from build123d import *

# Parameters (mm, degrees)
SKETCH1_W           = 50
SKETCH1_H           = 50
BOSS_EXTRUDE1_DEPTH = 3
BOSS_EXTRUDE2_DEPTH = 6
CUT_EXTRUDE1_DEPTH  = 2.1
CUT_EXTRUDE2_DEPTH  = 2.5
CUT_EXTRUDE3_DEPTH  = 3.3
SKETCH4_R           = 1.55
SKETCH4_R_2         = 1.8
SKETCH4_R_3         = 2.4
CUT_EXTRUDE4_DEPTH  = 37.482872694
CUT_EXTRUDE5_REACH  = 38.483
SKETCH5_W           = 3.1
SKETCH5_H           = 6
SKETCH5_W_2         = 6
SKETCH5_H_2         = 3.6
SKETCH5_W_3         = 4.8


with BuildPart() as part:
    # Sketch1 → Boss-Extrude1 (new body)
    with BuildSketch(Plane(origin=(0, 0, 0), x_dir=(1, 0, 0), z_dir=(0, 1, 0))):
        Rectangle(SKETCH1_W, SKETCH1_H)
    extrude(amount=BOSS_EXTRUDE1_DEPTH)

    # Sketch2 → Boss-Extrude2 (add)
    with BuildSketch(Plane(origin=(0, 3, 0), x_dir=(1, 0, 0), z_dir=(0, 1, 0))):
        Polygon((-13, 13), (-25, 13), (-25, 25), (25, 25), (25, -25), (-25, -25), (-25, -13), (-13, -13), (13, -13), (13, 13), align=None)
    extrude(amount=BOSS_EXTRUDE2_DEPTH)

    # Sketch3 → Cut-Extrude1 (cut)
    with BuildSketch(Plane(origin=(0, 3, 0), x_dir=(1, 0, 0), z_dir=(0, 1, 0))):
        Polygon((-21.5, 25), (-16.5, 25), (-16.5, 20.443375673), (-16.5, 17.556624327), (-19, 16.113248654), (-21.5, 17.556624327), (-21.5, 20.443375673), align=None)
        Polygon((-8.55, 25), (-3.45, 25), (-3.45, 20.472243186), (-3.45, 17.527756814), (-6, 16.055513627), (-8.55, 17.527756814), (-8.55, 20.472243186), align=None)
        Polygon((4.4, 25), (9.6, 25), (9.6, 20.5011107), (9.6, 17.4988893), (7, 15.9977786), (4.4, 17.4988893), (4.4, 20.5011107), align=None)
    extrude(amount=CUT_EXTRUDE1_DEPTH, mode=Mode.SUBTRACT)

    # Sketch3<3> → Cut-Extrude2 (cut)
    with BuildSketch(Plane(origin=(0, 3, 0), x_dir=(1, 0, 0), z_dir=(0, 1, 0))):
        Polygon((25, 15.75), (25, 10.25), (20.58771324, 10.25), (17.41228676, 10.25), (15.824573519, 13), (17.41228676, 15.75), (20.58771324, 15.75), align=None)
        Polygon((25, 2.8), (25, -2.8), (20.616580754, -2.8), (17.383419246, -2.8), (15.766838493, 0), (17.383419246, 2.8), (20.616580754, 2.8), align=None)
        Polygon((25, -10.15), (25, -15.85), (20.645448267, -15.85), (17.354551733, -15.85), (15.709103466, -13), (17.354551733, -10.15), (20.645448267, -10.15), align=None)
    extrude(amount=CUT_EXTRUDE2_DEPTH, mode=Mode.SUBTRACT)

    # Sketch3<4> → Cut-Extrude3 (cut)
    with BuildSketch(Plane(origin=(0, 3, 0), x_dir=(1, 0, 0), z_dir=(0, 1, 0))):
        Polygon((-22.6, -21.078460969), (-22.6, -25), (-15.4, -25), (-15.4, -21.078460969), (-15.4, -16.921539031), (-19, -14.843078062), (-22.6, -16.921539031), align=None)
        Polygon((-9.55, -21.049593456), (-9.55, -25), (-2.45, -25), (-2.45, -21.049593456), (-2.45, -16.950406544), (-6, -14.900813089), (-9.55, -16.950406544), align=None)
        Polygon((3.5, -21.020725942), (3.5, -25), (10.5, -25), (10.5, -21.020725942), (10.5, -16.979274058), (7, -14.958548116), (3.5, -16.979274058), align=None)
    extrude(amount=CUT_EXTRUDE3_DEPTH, mode=Mode.SUBTRACT)

    # Sketch4 → Cut-Extrude4 (cut, through all)
    with BuildSketch(Plane(origin=(0, 9, 0), x_dir=(1, 0, 0), z_dir=(0, 1, 0))):
        with Locations(Location((-19, 19, 0), (0, 0, 270))):
            Circle(SKETCH4_R)
        with Locations(Location((-6, 19, 0), (0, 0, 270))):
            Circle(SKETCH4_R)
        with Locations(Location((7, 19, 0), (0, 0, 270))):
            Circle(SKETCH4_R)
        with Locations(Location((19, 13, 0), (0, 0, 270))):
            Circle(SKETCH4_R_2)
        with Locations(Location((19, 0, 0), (0, 0, 270))):
            Circle(SKETCH4_R_2)
        with Locations(Location((19, -13, 0), (0, 0, 270))):
            Circle(SKETCH4_R_2)
        with Locations(Location((7, -19, 0), (0, 0, 270))):
            Circle(SKETCH4_R_3)
        with Locations(Location((-6, -19, 0), (0, 0, 270))):
            Circle(SKETCH4_R_3)
        with Locations(Location((-19, -19, 0), (0, 0, 270))):
            Circle(SKETCH4_R_3)
    extrude(amount=-CUT_EXTRUDE4_DEPTH, mode=Mode.SUBTRACT)

    # Cut-Extrude5: up to this face of the body (flat: up to its plane)
    cut_extrude5_end = Plane(part.part.faces().sort_by_distance((-19, 3, 24.875499774))[0])
    # Sketch5 → Cut-Extrude5 (cut, up to the picked face)
    with BuildSketch(Plane(origin=(0, 9, 0), x_dir=(1, 0, 0), z_dir=(0, 1, 0)), mode=Mode.PRIVATE) as cut_extrude5_sk1:
        with Locations((-19, 22)):
            Rectangle(SKETCH5_W, SKETCH5_H)
    cut_extrude5_tool1 = split(extrude(cut_extrude5_sk1.sketch, amount=-CUT_EXTRUDE5_REACH, mode=Mode.PRIVATE), bisect_by=cut_extrude5_end, keep=Keep.BOTH, mode=Mode.PRIVATE)
    # Sketch5 → Cut-Extrude5 (cut, up to the picked face)
    with BuildSketch(Plane(origin=(0, 9, 0), x_dir=(1, 0, 0), z_dir=(0, 1, 0)), mode=Mode.PRIVATE) as cut_extrude5_sk2:
        with Locations((-6, 22)):
            Rectangle(SKETCH5_W, SKETCH5_H)
    cut_extrude5_tool2 = split(extrude(cut_extrude5_sk2.sketch, amount=-CUT_EXTRUDE5_REACH, mode=Mode.PRIVATE), bisect_by=cut_extrude5_end, keep=Keep.BOTH, mode=Mode.PRIVATE)
    # Sketch5 → Cut-Extrude5 (cut, up to the picked face)
    with BuildSketch(Plane(origin=(0, 9, 0), x_dir=(1, 0, 0), z_dir=(0, 1, 0)), mode=Mode.PRIVATE) as cut_extrude5_sk3:
        with Locations((7, 22)):
            Rectangle(SKETCH5_W, SKETCH5_H)
    cut_extrude5_tool3 = split(extrude(cut_extrude5_sk3.sketch, amount=-CUT_EXTRUDE5_REACH, mode=Mode.PRIVATE), bisect_by=cut_extrude5_end, keep=Keep.BOTH, mode=Mode.PRIVATE)
    # Sketch5 → Cut-Extrude5 (cut, up to the picked face)
    with BuildSketch(Plane(origin=(0, 9, 0), x_dir=(1, 0, 0), z_dir=(0, 1, 0)), mode=Mode.PRIVATE) as cut_extrude5_sk4:
        with Locations((22, 13)):
            Rectangle(SKETCH5_W_2, SKETCH5_H_2)
    cut_extrude5_tool4 = split(extrude(cut_extrude5_sk4.sketch, amount=-CUT_EXTRUDE5_REACH, mode=Mode.PRIVATE), bisect_by=cut_extrude5_end, keep=Keep.BOTH, mode=Mode.PRIVATE)
    # Sketch5 → Cut-Extrude5 (cut, up to the picked face)
    with BuildSketch(Plane(origin=(0, 9, 0), x_dir=(1, 0, 0), z_dir=(0, 1, 0)), mode=Mode.PRIVATE) as cut_extrude5_sk5:
        with Locations((22, 0)):
            Rectangle(SKETCH5_W_2, SKETCH5_H_2)
    cut_extrude5_tool5 = split(extrude(cut_extrude5_sk5.sketch, amount=-CUT_EXTRUDE5_REACH, mode=Mode.PRIVATE), bisect_by=cut_extrude5_end, keep=Keep.BOTH, mode=Mode.PRIVATE)
    # Sketch5 → Cut-Extrude5 (cut, up to the picked face)
    with BuildSketch(Plane(origin=(0, 9, 0), x_dir=(1, 0, 0), z_dir=(0, 1, 0)), mode=Mode.PRIVATE) as cut_extrude5_sk6:
        with Locations((22, -13)):
            Rectangle(SKETCH5_W_2, SKETCH5_H_2)
    cut_extrude5_tool6 = split(extrude(cut_extrude5_sk6.sketch, amount=-CUT_EXTRUDE5_REACH, mode=Mode.PRIVATE), bisect_by=cut_extrude5_end, keep=Keep.BOTH, mode=Mode.PRIVATE)
    # Sketch5 → Cut-Extrude5 (cut, up to the picked face)
    with BuildSketch(Plane(origin=(0, 9, 0), x_dir=(1, 0, 0), z_dir=(0, 1, 0)), mode=Mode.PRIVATE) as cut_extrude5_sk7:
        with Locations((7, -22)):
            Rectangle(SKETCH5_W_3, SKETCH5_H)
    cut_extrude5_tool7 = split(extrude(cut_extrude5_sk7.sketch, amount=-CUT_EXTRUDE5_REACH, mode=Mode.PRIVATE), bisect_by=cut_extrude5_end, keep=Keep.BOTH, mode=Mode.PRIVATE)
    # Sketch5 → Cut-Extrude5 (cut, up to the picked face)
    with BuildSketch(Plane(origin=(0, 9, 0), x_dir=(1, 0, 0), z_dir=(0, 1, 0)), mode=Mode.PRIVATE) as cut_extrude5_sk8:
        with Locations((-6, -22)):
            Rectangle(SKETCH5_W_3, SKETCH5_H)
    cut_extrude5_tool8 = split(extrude(cut_extrude5_sk8.sketch, amount=-CUT_EXTRUDE5_REACH, mode=Mode.PRIVATE), bisect_by=cut_extrude5_end, keep=Keep.BOTH, mode=Mode.PRIVATE)
    # Sketch5 → Cut-Extrude5 (cut, up to the picked face)
    with BuildSketch(Plane(origin=(0, 9, 0), x_dir=(1, 0, 0), z_dir=(0, 1, 0)), mode=Mode.PRIVATE) as cut_extrude5_sk9:
        with Locations((-19, -22)):
            Rectangle(SKETCH5_W_3, SKETCH5_H)
    cut_extrude5_tool9 = split(extrude(cut_extrude5_sk9.sketch, amount=-CUT_EXTRUDE5_REACH, mode=Mode.PRIVATE), bisect_by=cut_extrude5_end, keep=Keep.BOTH, mode=Mode.PRIVATE)
    add(cut_extrude5_tool1.solids().sort_by(Axis((-19, 9, -22), (0, -1, 0)))[0], mode=Mode.SUBTRACT)
    add(cut_extrude5_tool2.solids().sort_by(Axis((-6, 9, -22), (0, -1, 0)))[0], mode=Mode.SUBTRACT)
    add(cut_extrude5_tool3.solids().sort_by(Axis((7, 9, -22), (0, -1, 0)))[0], mode=Mode.SUBTRACT)
    add(cut_extrude5_tool4.solids().sort_by(Axis((22, 9, -13), (0, -1, 0)))[0], mode=Mode.SUBTRACT)
    add(cut_extrude5_tool5.solids().sort_by(Axis((22, 9, 0), (0, -1, 0)))[0], mode=Mode.SUBTRACT)
    add(cut_extrude5_tool6.solids().sort_by(Axis((22, 9, 13), (0, -1, 0)))[0], mode=Mode.SUBTRACT)
    add(cut_extrude5_tool7.solids().sort_by(Axis((7, 9, 22), (0, -1, 0)))[0], mode=Mode.SUBTRACT)
    add(cut_extrude5_tool8.solids().sort_by(Axis((-6, 9, 22), (0, -1, 0)))[0], mode=Mode.SUBTRACT)
    add(cut_extrude5_tool9.solids().sort_by(Axis((-19, 9, 22), (0, -1, 0)))[0], mode=Mode.SUBTRACT)


solid = part.part
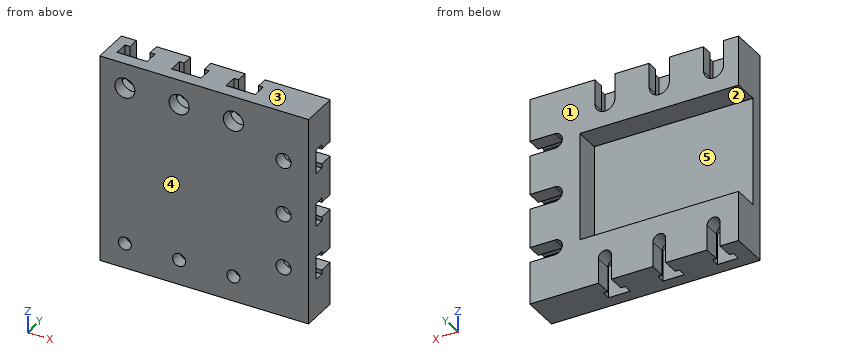
Input: part model. Units: mm. Frame: model coordinates. Face numbers are marked on the shaded views. A direction names the side the tool comes from. Give positions to 0.01 mm unless a question says otherwise; leave off trailing zeros. Loops run counter-clockwise (first coordinate to the right, second up) from the corner with the lowest first, then second, coordinate; pieces in that order, holes last. Notation, with made-up numbers: M 40,54.5 L 87,54.5 A19 ccw 87,66.5 Z; hole C 60,-31 d10. An arc over 180 degrees is marked long. Use CSV: the item, a comma, the result in double quotes.
(1) Set-up query: the marked faces 1 and 2. Return all of +Z, -Z, +X, -X, +Y, -Y with unobstructed straight access to the full face (end or side cutting, diameter ignored); none if empty.
Outcome:
face 1,"+Z, -Z, +X, -X, +Y"
face 2,"-X, +Y"
(2) Pin query (flat end, axial travel): P1, Ø13, axis at x = -9, z = -2, coming from the +Y side. Return the tip coordinate at first contact, or that it passes through.
Outcome:
P1,"stops at y = 3"
(3) Pull-direction query (Z, two-part tool) for the marked faces 3, 4 and 5; classes: pulls with the +Z half, pulls with the -Z half, needs draft (parallel to the pull), parting line crosses it, or undercut.
Outcome:
face 3,"pulls with the +Z half"
face 4,"needs draft"
face 5,"undercut"
(4) Section C-C, the plane z = -21.5. Return loops of the section in (x, y), plus the area to 3 significant figures.
Outcome:
outline,"M -25,0 L 25,0 L 25,9 L 8.55,9 L 8.55,5.1 L 9.6,5.1 L 9.6,3 L 4.4,3 L 4.4,5.1 L 5.45,5.1 L 5.45,9 L -4.45,9 L -4.45,5.1 L -3.45,5.1 L -3.45,3 L -8.55,3 L -8.55,5.1 L -7.55,5.1 L -7.55,9 L -17.45,9 L -17.45,5.1 L -16.5,5.1 L -16.5,3 L -21.5,3 L -21.5,5.1 L -20.55,5.1 L -20.55,9 L -25,9 Z"
area,"382 mm²"
(5) Section B-B, the plane x = 1. Return loops of the section in (y, z).
Outcome:
outline,"M 0,-25 L 9,-25 L 9,-13 L 3,-13 L 3,13 L 9,13 L 9,25 L 0,25 Z"
(6) Material intervals for L1, parallel to Z at x = 20, y = 7; L2, parallel to X at y = 1.8, z = -19; L3, parallel to Y at x = -15.5, z = 21.5, sorted ascending. Write a range as [from, to].
Outcome:
L1,"z = [-25, -14.8], [-11.2, -1.8], [1.8, 11.2], [14.8, 25]"
L2,"x = [-25, -20.55], [-17.45, -7.55], [-4.45, 5.45], [8.55, 25]"
L3,"y = [0, 3], [6.3, 9]"
(7) Section D-D, the plane z = 6.5. Return loops of the section in (x, y).
Outcome:
outline,"M -25,0 L 25,0 L 25,9 L 13,9 L 13,3 L -25,3 Z"
(8) Section A-A, the plane y = 1.5. Count the separate pieces of the cut face and the enclosed holes in it, plus the area to 3 significant figures.
Outcome:
separate pieces,"1"
enclosed holes,"9"
area,"2,390 mm²"
